Source: three-view drawing plus pictorial views. Frame: mm from the lowest corner of the part. A direction names the side the tool comes from. Round coordinates to 2 decimals unless told otherwise and drop trailing zeros. Loops run counter-clockwise (first coordinate to the right, second up) from the corner with the lowest first, then second, coordinate; pieces in that order, holes last. Notation, with made-up numbers: (23.5, -19) -> (62.5, -19) arc R37 ccw to (62.5, 19) -> close; hole circle Ø10 at (72, -22.5). An arc over 180 degrees is marked (long way). Answer as a JSON object with one key per item and string values. Group by question number.
Item 1: Pin query (flat end, axial travel): pin 1 (11.5 mm diameter, centred on x = 12, y = 15, fed in from +Z); pin 2 (5.5 mm diameter, centred on x = 88, y = 55, fed in from -Z); pin 3 (2.5 mm diameter, centred on x = 35, z = 13.5, fed in from +Y). Return the tip coordinate at first contact, or that it passes through.
Item 2: Material intervals for line 1 (Y direction, x = 88, z = 2.75); line 2 (Y direction, x = 6, z = 13.5); line 3 (X direction, y = 31, z = 1.75), sorted ascending. Write a range as [from, to].
Item 3: Section query A-A on x = 53.5. Return loops of the section in (y, z).
Item 4: Section query B-B on z = 1.5. Return loops of the section in (x, y).
Item 5: Section query C-C on y = 15. Return loops of the section in (x, z), and give its area (3 significant figures).
Item 6: Draft query along X for the marked faces 4, 5 and 6. Return one class per face: released by +X, released by -X, zero draft, split by the parting line, or undercut.
Item 7: Section query D-D on y = 28.5. Return loops of the section in (x, z).
Item 8: Set-up query: the marked faces 1, 2 and 3. Return all of +Z, -Z, +X, -X, +Y, -Y with unobstructed straight access to the full face (end or side cutting, diameter ignored); none if empty.
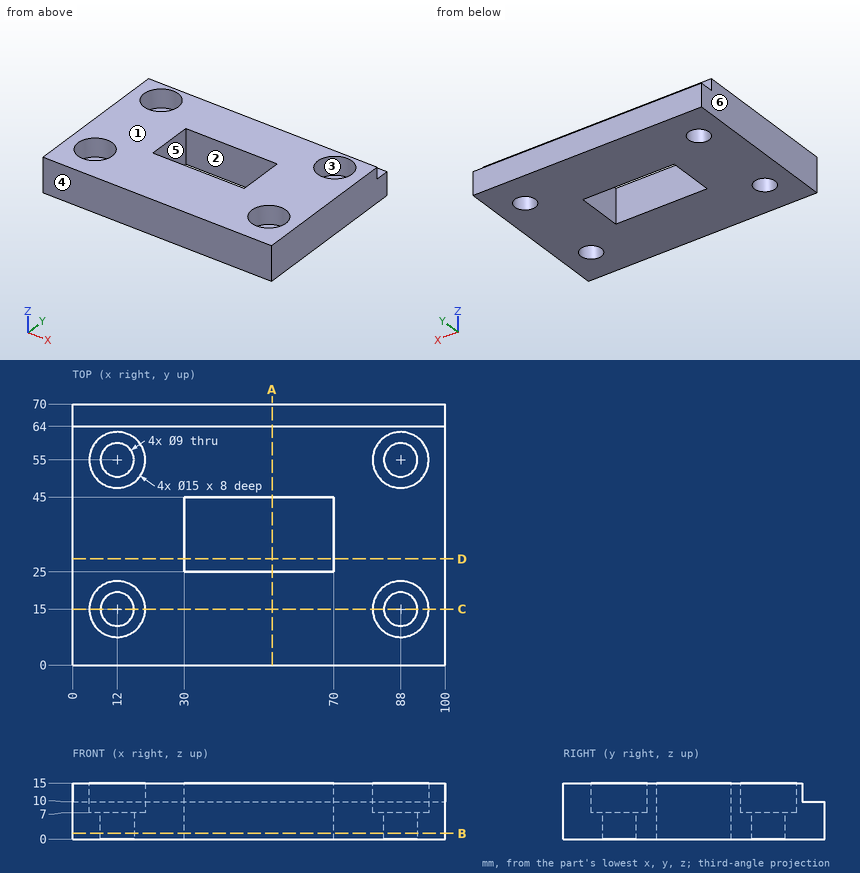
Solved:
{
 "1": {"pin 1": "z = 7", "pin 2": "through", "pin 3": "y = 64"},
 "2": {"line 1": "[0, 10.5], [19.5, 50.5], [59.5, 70]", "line 2": "[0, 10.5], [19.5, 50.5], [59.5, 64]", "line 3": "[0, 30], [70, 100]"},
 "3": {"outline": "(0, 0) -> (25, 0) -> (25, 15) -> (0, 15) -> close; (45, 0) -> (70, 0) -> (70, 10) -> (64, 10) -> (64, 15) -> (45, 15) -> close"},
 "4": {"outline": "(0, 0) -> (100, 0) -> (100, 70) -> (0, 70) -> close; hole circle Ø9 at (12, 15); hole circle Ø9 at (12, 55); hole (30, 25) -> (70, 25) -> (70, 45) -> (30, 45) -> close; hole circle Ø9 at (88, 15); hole circle Ø9 at (88, 55)"},
 "5": {"outline": "(0, 0) -> (7.5, 0) -> (7.5, 7) -> (4.5, 7) -> (4.5, 15) -> (0, 15) -> close; (16.5, 0) -> (83.5, 0) -> (83.5, 7) -> (80.5, 7) -> (80.5, 15) -> (19.5, 15) -> (19.5, 7) -> (16.5, 7) -> close; (92.5, 0) -> (100, 0) -> (100, 15) -> (95.5, 15) -> (95.5, 7) -> (92.5, 7) -> close", "area": "1,130 mm²"},
 "6": {"face 4": "zero draft", "face 5": "undercut", "face 6": "released by -X"},
 "7": {"outline": "(0, 0) -> (30, 0) -> (30, 15) -> (0, 15) -> close; (70, 0) -> (100, 0) -> (100, 15) -> (70, 15) -> close"},
 "8": {"face 1": "+Z, +X, -X, +Y, -Y", "face 2": "+Z, -Z", "face 3": "+Z"}
}
